```python
from build123d import *

# Parameters (mm, degrees)
F0_W     = 26
F0_H     = 17
F1_DEPTH = 16
F2_W     = 23
F2_H     = 15.5
F3_DEPTH = 14.5
F5_DEPTH = 25


with BuildPart() as f1:
    # F0 (on Front) → F1 (new body)
    with BuildSketch(Plane.XZ):
        with Locations((13, 8.5)):
            Rectangle(F0_W, F0_H)
    extrude(amount=-F1_DEPTH)

    # F2 (on Front) → F3 (cut)
    with BuildSketch(Plane.XZ):
        with Locations((13, 7.75)):
            Rectangle(F2_W, F2_H)
    extrude(amount=-F3_DEPTH, mode=Mode.SUBTRACT)

    # F4 (on Front) → F5 (cut)
    with BuildSketch(Plane.XZ):
        with BuildLine():
            Line((14.5, 0), (14.5, 5))
            ThreePointArc((14.5, 5), (13, 6.5), (11.5, 5))
            Line((11.5, 5), (11.5, 0))
            Line((11.5, 0), (14.5, 0))
        make_face()
    extrude(amount=-F5_DEPTH, mode=Mode.SUBTRACT)


solid = f1.part
```
Can you work these out from the model? Positions are in its coordinate system, mm. A direction names the side the tool comes from. Coordinates: 2 decimals unless noted, no trailing zeros. Order: outer loops, then holes, each group sorted by start corner. A loop starts at its lowest first (then second) coordinate and runs counter-clockwise, first axis right, second up.
1. I need wall thicknesses on line 1 (X direction, y = 11, z = 5); line 2 (Y direction, x = 20.75, z = 7.75); line 3 (Z direction, x = 21, y = 4). Which ranges of each line are inside material? Lowest first, please.
2. If we section it at C-C (y = 5): Please give me the cut outline in (x, z), then the cut area to 3 significant figures.
3. Thinking about a two-plate mould opening in X: for faces 1 (the face through (0, 8, 8)), 2 (the face through (14.5, 15, 2)), 3 (the face through (1, 10, 0)), which applies, +X half, -X half, draft (parallel to the pull), parting line (faces both ways), or undercut?
4. If we section it at A-A (x = 13): Please give me the cut outline in (y, z), then the cut area to 3 significant figures.
5. If we section it at B-B (z = 11.25): Please give me the cut outline in (x, y).
6. I'm going to push flat-ended pins straight in: pin 1 (7 mm diameter, centred on x = 12, y = 10.5, fed in from -Z); pin 2 (4.5 mm diameter, centred on x = 16, z = 10, fed in from -Y). Where does each tip first touch, or does it pass through?
7. For faces 4 (the face through (10, 0, 16)), 5 (the face through (11.5, 15, 3)), 6 (the face through (1.5, 7, 8)), which set-ups out of +Z, -Z, +X, -X, +Y, -Y let a thin tool reach every point of the face, with its end or its side?
8. If we section it at D-D (x = 23.5): Please give me the cut outline in (y, z).
Entries:
1. line 1: x = 0 to 1.5, 24.5 to 26
1. line 2: y = 14.5 to 16
1. line 3: z = 15.5 to 17
2. outline: (0, 0) - (1.5, 0) - (1.5, 15.5) - (24.5, 15.5) - (24.5, 0) - (26, 0) - (26, 17) - (0, 17) - close
2. area: 85.5 mm2
3. face 1: -X half
3. face 2: undercut
3. face 3: draft
4. outline: (0, 15.5) - (14.5, 15.5) - (14.5, 6.5) - (16, 6.5) - (16, 17) - (0, 17) - close
4. area: 37.5 mm2
5. outline: (0, 0) - (1.5, 0) - (1.5, 14.5) - (24.5, 14.5) - (24.5, 0) - (26, 0) - (26, 16) - (0, 16) - close
6. pin 1: stops at z = 15.5
6. pin 2: stops at y = 14.5
7. face 4: +Z, -Z, +X, -X, -Y
7. face 5: -Z, +Y, -Y
7. face 6: -Z, -Y
8. outline: (0, 15.5) - (14.5, 15.5) - (14.5, 0) - (16, 0) - (16, 17) - (0, 17) - close
